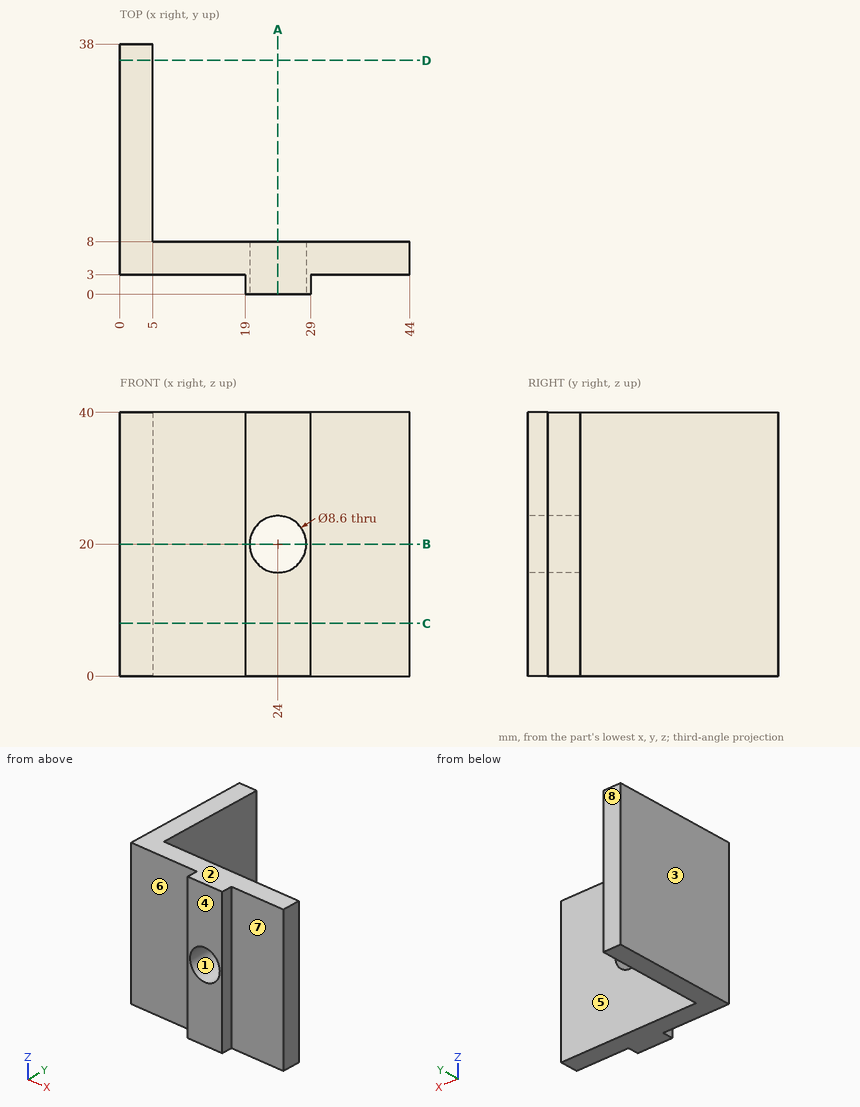
Job drawing, mm, ordinate dimensions from the low corner. One solid piece. A direction names the side the tool comes from. Coordinates: 2 decimals unless noted, no trailing zeros. Write each loop counter-clockwise with the first axis right and the second up, starting at its lowest first coordinate (ties: lowest second). Pieces come first, ordered by that corner, then holes.
Item 1: Pin check, flat tips, straight feed: pin 1 (3 mm diameter, centred on y = 11.5, z = 22, fed in from +X); pin 2 (9.5 mm diameter, centred on x = 8.5, z = 20.5, fed in from -Y); pin 3 (2.5 mm diameter, centred on y = 1, z = 26.5, fed in from +X). Stop position of each tip, or through.
Item 2: Slice it at B-B (z = 20). Write the cut outline in (x, y), and give its area (3 significant figures).
Item 3: Slice it at D-D (y = 35.5). Write the cut outline in (x, z).
Item 4: Slice it at A-A (x = 24). Write the cut outline in (y, z).
Item 5: Slice it at C-C (z = 8). Write the cut outline in (x, y), and give its area (3 significant figures).
Item 6: Which spindle directions (+Z, -Z, +X, -X, +Y, -Y) get a long thin tool onto all of the face, cutting with end or side? Do the marked faces 4, 5, 6, 7 and 8. Say none if no direction does.
Item 7: Mould opens along X. For the marked faces 1, 2 and 3 say: released by +X, released by -X, zero draft, split by the parting line, or undercut.
Item 8: Probe line 1 (Z direction, x = 24, y = 6.25); line 2 (X direction, y = 4, z = 20); line 3 (X direction, y = 2, z = 20). List the from-to ranges inside material, lowest first.
Results found:
1. pin 1: stops at x = 5
1. pin 2: stops at y = 3
1. pin 3: stops at x = 29
2. outline: (0, 3) - (19, 3) - (19, 0) - (19.7, 0) - (19.7, 8) - (5, 8) - (5, 38) - (0, 38) - close; (28.3, 0) - (29, 0) - (29, 3) - (44, 3) - (44, 8) - (28.3, 8) - close
2. area: 331 mm2
3. outline: (0, 0) - (5, 0) - (5, 40) - (0, 40) - close
4. outline: (0, 0) - (8, 0) - (8, 15.7) - (0, 15.7) - close; (0, 24.3) - (8, 24.3) - (8, 40) - (0, 40) - close
5. outline: (0, 3) - (19, 3) - (19, 0) - (29, 0) - (29, 3) - (44, 3) - (44, 8) - (5, 8) - (5, 38) - (0, 38) - close
5. area: 400 mm2
6. face 4: +Z, -Z, +X, -X, -Y
6. face 5: +Z, -Z, +X, +Y
6. face 6: +Z, -Z, -X, -Y
6. face 7: +Z, -Z, +X, -Y
6. face 8: +Z, -Z, +X, -X, +Y
7. face 1: undercut
7. face 2: zero draft
7. face 3: released by -X
8. line 1: z = 0 to 15.7, 24.3 to 40
8. line 2: x = 0 to 19.7, 28.3 to 44
8. line 3: x = 19 to 19.7, 28.3 to 29
